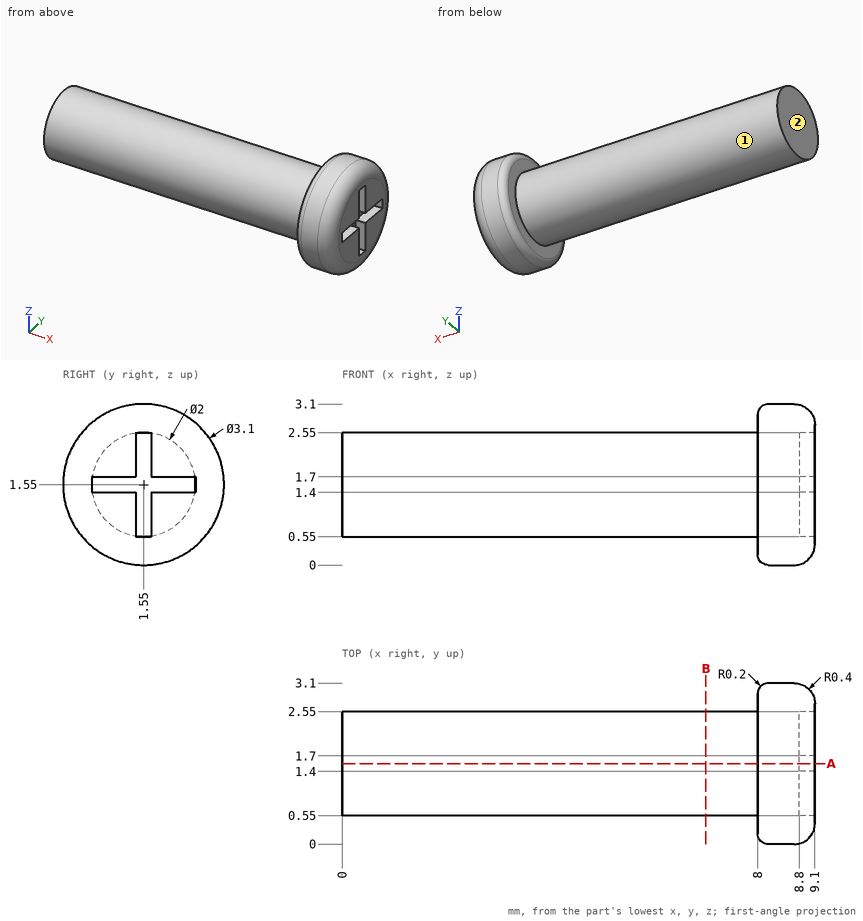
Geometry check sheet. Reference: drawing and pictorial views, mm from the part's lowest x, y, z. A direction names the side the tool comes from. Give positions to 0.01 mm unless a question says otherwise; leave off trailing zeros. Order: outer loops, then holes, each group sorted by start corner. A loop starts at its lowest first (then second) coordinate and runs counter-clockwise, first axis right, second up. Notation, with made-up numbers: (-13, -31.5) -> (20, -31.5) arc R24 cw to (20, -11.5) -> close; hole circle Ø3 at (24.5, 41.5). An arc over 180 degrees is marked (long way). Write each question's results on one line, items separated by ' | '. Start each with the question number.
(1) Gauge pin test, flat end, axial feed: P1, Ø1, axis at y = 2, z = 2.5, coming from the -X side. Record the tip position at first contact, or that the pin passes through.
(2) Sectioned sample at A-A (y = 1.55). Enter the section's corners in (x, z), plus the area to 3 significant figures.
(3) Scan lines: line 1 (X direction, y = 1.6, z = 1.1); line 2 (Y direction, x = 5, z = 1.35); line 3 (Y direction, x = 4, z = 0.75). Record each from-to range of solid material in increasing order.
(4) Access from +Z, -Z, +X, -X, +Y, -Y to the whole of each face (thin tool, end or side, straight path). Record for the marked faces 1 and 2.
(5) Sectioned sample at B-B (x = 7). Enter the section's corners in (y, z), plus the area to 3 significant figures.
Answer below:
1) P1: x = 0
2) outline: (0, 0.55) -> (8, 0.55) -> (8, 0.2) arc R0.2 ccw to (8.2, 0) -> (8.7, 0) arc R0.4 ccw to (9.1, 0.4) -> (9.1, 0.55) -> (8.8, 0.55) -> (8.8, 2.55) -> (9.1, 2.55) -> (9.1, 2.7) arc R0.4 ccw to (8.7, 3.1) -> (8.2, 3.1) arc R0.2 ccw to (8, 2.9) -> (8, 2.55) -> (0, 2.55) -> close | area: 18.7 mm2
3) line 1: 0 to 8.8 | line 2: 0.57 to 2.53 | line 3: 0.95 to 2.15
4) face 1: -X | face 2: +Z, -Z, -X, +Y, -Y
5) outline: circle Ø2 at (1.55, 1.55) | area: 3.14 mm2
